Geometry check sheet. Reference: the model listing, model coordinates, mm. Give positions to 0.01 mm unless a question says otherwise; leave off trailing zeros. Write each loop counter-clockwise with the first axis right and the second up, starting at its lowest first coordinate (ties: lowest second). Pieces come first, ordered by that corner, then holes. Notation, with made-up numbers: (-3, 1.25) -> (54, 1.25) arc R28 cw to (54, 31.25) -> close; hole circle Ø4 at (-5, 68.5). An arc over 180 degrees is marked (long way). Write item = value, one per line. Start each with the question number.
1. Cross-section at B-B, the plane z = 33.5. Record the cut outline in (x, y).
2. Thickness scan on line 1 along X through (y, z) = (35.5, 22); line 2 along X through (y, z) = (25, 27.5); line 3 along Y through (x, z) = (23, 27.5). Record the ranges inside material, lowest first.
3. Cross-section at A-A, the plane z = 10. Record the cut outline in (x, y).
4. Depth check by flat-ended pin: P1, Ø8, axis at x = 90, y = -2.5, coming from the -Z side; P2, Ø3, axis at y = -41.5, z = 27.5, coming from the -X side; P3, Ø3, axis at y = -40, z = 17.5, coming from the -X side; P4, Ø2, axis at x = 93, z = 10, coming from the +Y side. Enter the tip coordinate at first touch or a pass-through.
```python
from build123d import *

# Parameters (mm, degrees)
F1_DEPTH = 35
F2_SIZE  = 5


with BuildPart() as f1:
    # F0 (on Top) → F1 (new body)
    with BuildSketch(Plane.XY):
        with BuildLine():
            Line((88.641453, 39.457253), (38.641453, 39.457253))
            ThreePointArc((38.641453, 39.457253), (24.499317, 33.599388), (18.641453, 19.457253))
            Line((18.641453, 19.457253), (18.641453, -30.542747))
            ThreePointArc((18.641453, -30.542747), (24.499317, -44.684883), (38.641453, -50.542747))
            Line((38.641453, -50.542747), (88.641453, -50.542747))
            ThreePointArc((88.641453, -50.542747), (102.783589, -44.684883), (108.641453, -30.542747))
            Line((108.641453, -30.542747), (108.641453, 19.457253))
            ThreePointArc((108.641453, 19.457253), (102.783589, 33.599388), (88.641453, 39.457253))
        make_face()
    extrude(amount=F1_DEPTH)

    # F2
    f2_edges = [f1.edges().sort_by_distance(p)[0] for p in [
        (18.641453, -5.542747, 35),
    ]]
    chamfer(f2_edges, length=F2_SIZE)


solid = f1.part
```
Answers:
q1.outline = (22.14, -30.54) arc R16.5 ccw to (38.64, -47.04) -> (88.64, -47.04) arc R16.5 ccw to (105.14, -30.54) -> (105.14, 19.46) arc R16.5 ccw to (88.64, 35.96) -> (38.64, 35.96) arc R16.5 ccw to (22.14, 19.46) -> close
q2.line_1 = 26.7 to 100.58
q2.line_2 = 19.42 to 107.86
q2.line_3 = -43.01 to 31.92
q3.outline = (18.64, -30.54) arc R20 ccw to (38.64, -50.54) -> (88.64, -50.54) arc R20 ccw to (108.64, -30.54) -> (108.64, 19.46) arc R20 ccw to (88.64, 39.46) -> (38.64, 39.46) arc R20 ccw to (18.64, 19.46) -> close
q4.P1 = 0
q4.P2 = 21.02
q4.P3 = 20.29
q4.P4 = 39.17
